Autodesk Inventor part; units mm, degrees
ref_plane "YZ Plane" through (0, 0, 0) normal (1, 0, 0) x (0, 1, 0)
ref_plane "XZ Plane" through (0, 0, 0) normal (0, 1, 0) x (-1, 0, 0)
ref_plane "XY Plane" through (0, 0, 0) normal (0, 0, 1) x (1, 0, 0)
sketch "Sketch1" plane through (0, 0, 0) normal (0, 1, 0) x (-1, 0, 0)
  line L0 (0, 0) -> (29, 0)
  line L1 (29, 0) -> (29, 49)
  line L2 (29, 49) -> (0, 49)
  line L3 (0, 49) -> (0, 0)
  dimension "d0" = 49
  dimension "d1" = 29
extrude "Extrusion1" add sketch "Sketch1" along normal blind 6
sketch "Sketch2" plane through (0, 0, 0) normal (0, -1, 0) x (1, 0, 0)
  line L0 (-21.7451, 36.3583) -> (64.7541, 36.3583) construction
  line L1 (64.7541, 36.3583) -> (64.7541, 15.5155) construction
  line L2 (64.7541, 15.5155) -> (-21.7451, 15.5155) construction
  line L3 (-21.7451, 15.5155) -> (-21.7451, 36.3583) construction
  line L4 (-15.0514, 16.3583) -> (-15.0514, 33.992)
  line L5 (-15.0514, 33.992) -> (-21.7613, 33.992)
  line L6 (-21.7613, 33.992) -> (-21.7613, 36.3583)
  line L7 (-21.7613, 36.3583) -> (-5.6835, 36.3583)
  line L8 (-5.6835, 36.3583) -> (-5.6835, 33.992)
  line L9 (-5.6835, 33.992) -> (-12.3934, 33.992)
  line L10 (-12.3934, 33.992) -> (-12.3934, 16.3583)
  line L11 (-12.3934, 16.3583) -> (-15.0514, 16.3583)
  point P0 (0, 0)
emboss "Emboss1" sketch "Sketch2" operation cut depth 2 direction (0, 1, 0)
properties part number "pegshort" material "PET Plastic"
Here's how the part is built. I have some questions about the finished solid (model axes, mm). A direction names the side the tool comes from. Coordinates: 2 decimals unless noted, no trailing zeros. Write each loop counter-clockwise with the first axis right and the second up, starting at its lowest first coordinate (ties: lowest second). Pieces come first, ordered by that corner, then holes.
Item 1: I want a section at A-A on y = 1.45. Write out the boundary of the cut face in (x, z), and give its area (3 significant figures).
Item 2: I want a section at B-B on z = 25.5. Write out the boundary of the cut face in (x, y).
Item 3: If I drill on line 1 (Z direction, x = -8.5, y = 1.3); line 2 (Y direction, x = -14, z = 19.5), over which ranges is the centre line in solid material (lowest first)?
Item 4: On a 3-axis mill with a long thin cutter (end or side, diameter ignored), from which of +Z, -Z, +X, -X, +Y, -Y can I reach the whole of each face in a straight line? I mean faces 1 (the flat face through (-14, 1, 36.358)), 2 (the flat face through (-15, 3, 49)). Say none if no direction works.
Item 5: If we mould it in two halves opening along X, with no side actions, what happens to faces 3 (the flat face through (-18, 0, 25)), 4 (the flat face through (0, 3, 25)), 5 (the flat face through (-12.393, 1, 25))? For each: +X half, -X half, draft (parallel to the pull), parting line (faces both ways), or undercut.
Item 6: I want a section at C-C on x = -15.75. Write out the boundary of the cut face in (y, z), and give its area (3 significant figures).
Findings below:
1. outline: (-29, 0) - (0, 0) - (0, 49) - (-29, 49) - close; hole (-21.76, 33.99) - (-15.05, 33.99) - (-15.05, 16.36) - (-12.39, 16.36) - (-12.39, 33.99) - (-5.68, 33.99) - (-5.68, 36.36) - (-21.76, 36.36) - close
1. area: 1,340 mm2
2. outline: (-29, 0) - (-15.05, 0) - (-15.05, 2) - (-12.39, 2) - (-12.39, 0) - (0, 0) - (0, 6) - (-29, 6) - close
3. line 1: z = 0 to 33.99, 36.36 to 49
3. line 2: y = 2 to 6
4. face 1: -Y
4. face 2: +Z, +X, -X, +Y, -Y
5. face 3: draft
5. face 4: +X half
5. face 5: undercut
6. outline: (0, 0) - (6, 0) - (6, 49) - (0, 49) - (0, 36.36) - (2, 36.36) - (2, 33.99) - (0, 33.99) - close
6. area: 289 mm2
